Verification items for the finished model (mm, model axes). Face numbers are marked on the shaded views. A direction names the side the tool comes from. Give positions to 0.01 mm unless a question says otherwise; leave off trailing zeros. Order: outer loops, then holes, each group sorted by start corner. A loop starts at its lowest first (then second) coordinate and runs counter-clockwise, first axis right, second up. Notation, with made-up numbers: (8.25, 37) - (52.25, 37) arc R17 cw to (52.25, 63) - close; hole circle Ø9 at (-3.5, -26.75). An arc over 180 degrees is marked (long way). Answer as a JSON object with one key per item and string values.
```python
from build123d import *

# Parameters (mm, degrees)
SKETCH_1_R                       = 5
EXTRUDE_1_DEPTH                  = 20
SKETCH_3_W                       = 0.6
SKETCH_3_H                       = 3
EXTRUDE_2_DEPTH                  = 2
FILLET_1_R                       = 0.2
PATTERN_CIRCULAR_3_COUNT         = 16
FILLET_1_OF_PATTERN_CIRCULAR_3_R = 0.2
SKETCH_4_W                       = 5.353265718
SKETCH_4_H                       = 11.52836058
CUT_EXTRUDE_1_DEPTH              = 4


with BuildPart() as part:
    # 草图1 → 凸台-拉伸1 (new body)
    with BuildSketch(Plane(origin=(0, 0, 0), x_dir=(1, 0, 0), z_dir=(0, 1, 0))):
        Circle(SKETCH_1_R)
    extrude(amount=EXTRUDE_1_DEPTH)

    # 草图3 → 凸台-拉伸2 (add)
    with BuildSketch(Plane(origin=(1.423145242, 19.89821487, 0), x_dir=(0, 0, -1), z_dir=(0.071339025, 0.997452126, 0))):
        with Locations((0, -2.894865204)):
            Rectangle(SKETCH_3_W, SKETCH_3_H)
    extrude_2 = extrude(amount=EXTRUDE_2_DEPTH)

    # 圆角1
    fillet_1_edges = [part.edges().sort_by_distance(p)[0] for p in [
        (4.453312743, 21.686602261, -0.3),
        (4.453312743, 21.686602261, 0.3),
    ]]
    fillet(fillet_1_edges, radius=FILLET_1_R)

    # 阵列(圆周)3: 凸台-拉伸2 ×16 about axis
    pattern_circular_3_axis = Axis((0, 0, 0), (0, 1, 0))
    for i in range(1, PATTERN_CIRCULAR_3_COUNT):
        add(extrude_2.rotate(pattern_circular_3_axis, i * 360 / PATTERN_CIRCULAR_3_COUNT))

    # 圆角1 of 阵列(圆周)3
    fillet_1_of_pattern_circular_3_edges = [part.edges().sort_by_distance(p)[0] for p in [
        (3.999519466, 21.686602261, -1.981372866),
        (4.229129525, 21.686602261, -1.427045146),
        (2.936835605, 21.686602261, -3.361099674),
        (3.361099674, 21.686602261, -2.936835605),
        (1.427045146, 21.686602261, -4.229129525),
        (1.981372866, 21.686602261, -3.999519466),
        (-0.3, 21.686602261, -4.453312743),
        (0.3, 21.686602261, -4.453312743),
        (-1.981372866, 21.686602261, -3.999519466),
        (-1.427045146, 21.686602261, -4.229129525),
        (-3.361099674, 21.686602261, -2.936835605),
        (-2.936835605, 21.686602261, -3.361099674),
        (-4.229129525, 21.686602261, -1.427045146),
        (-3.999519466, 21.686602261, -1.981372866),
        (-4.453312743, 21.686602261, 0.3),
        (-4.453312743, 21.686602261, -0.3),
        (-3.999519466, 21.686602261, 1.981372866),
        (-4.229129525, 21.686602261, 1.427045146),
        (-2.936835605, 21.686602261, 3.361099674),
        (-3.361099674, 21.686602261, 2.936835605),
        (-1.427045146, 21.686602261, 4.229129525),
        (-1.981372866, 21.686602261, 3.999519466),
        (0.3, 21.686602261, 4.453312743),
        (-0.3, 21.686602261, 4.453312743),
        (1.981372866, 21.686602261, 3.999519466),
        (1.427045146, 21.686602261, 4.229129525),
        (3.361099674, 21.686602261, 2.936835605),
        (2.936835605, 21.686602261, 3.361099674),
        (4.229129525, 21.686602261, 1.427045146),
        (3.999519466, 21.686602261, 1.981372866),
    ]]
    fillet(fillet_1_of_pattern_circular_3_edges, radius=FILLET_1_OF_PATTERN_CIRCULAR_3_R)

    # 草图4 → 切除-拉伸1 (cut)
    with BuildSketch(Plane(origin=(0, 0, 0), x_dir=(-1, 0, 0), z_dir=(0, -1, 0))):
        Rectangle(SKETCH_4_W, SKETCH_4_H)
    extrude(amount=-CUT_EXTRUDE_1_DEPTH, mode=Mode.SUBTRACT)


solid = part.part
```
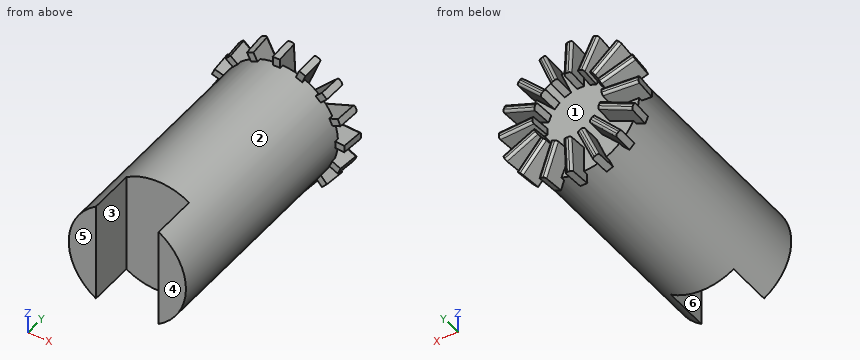
(1) Material ranges on line 1 along Y through (x, z) = (0.75, -1); line 2 along Y through (x, z) = (2.75, -2); line 3 along X through (y, z) = (3, -1.5), recorded low to high. Write a range as [from, to].
Computed values:
{"line 1": "y = [4, 20]", "line 2": "y = [0, 20]", "line 3": "x = [-4.77, -2.68], [2.68, 4.77]"}
(2) Section check A-A (y = 2.5). Record the cut outline in (x, z).
Computed values:
{"outline": "(-2.68, -4.22) - (-2.68, 4.22) arc R5 ccw to start; (2.68, -4.22) arc R5 ccw to (2.68, 4.22) - close"}
(3) Release check for a two-part mould opening along X. For the marked faces 5 and 6 record: pulls with the +X half, pulls with the -X half, needs draft (parallel to the pull), parting line crosses it, or undercut.
Computed values:
{"face 5": "needs draft", "face 6": "undercut"}
(4) Access from +Z, -Z, +X, -X, +Y, -Y to the whole of each face (thin tool, end or side, straight path). Record for the marked faces 1, 2, 3 and 4.
Computed values:
{"face 1": "+Y", "face 2": "-Y", "face 3": "+Z, -Z, -Y", "face 4": "+Z, -Z, +X, -X, -Y"}
(5) Section check B-B (y = 5). Record the cut outline in (x, z).
Computed values:
{"outline": "circle Ø10 at (0, 0)"}
(6) Gauge pin test, flat ends, axial feed: pin 1 Ø1.6 at (x, z) = (0.5, 1) entering from -Y; pin 2 Ø1 at (x, y) = (-0.5, 14) entering from +Z; pin 3 Ø2 at (y, z) = (20.5, -4.5) entering from +X. Record the tip position at first contact, or that the pin passes through.
Computed values:
{"pin 1": "stops at y = 4", "pin 2": "stops at z = 5", "pin 3": "stops at x = 4.41"}
